Read the model definition and answer for the solid it produces. Units are mm, in the model's axes. A direction names the side the tool comes from. Coordinates: 2 decimals unless noted, no trailing zeros. Order: outer loops, then holes, each group sorted by start corner. A loop starts at its lowest first (then second) coordinate and runs counter-clockwise, first axis right, second up. Notation, with made-up numbers: (-24.5, -26) - (-12.5, -26) arc R19 ccw to (-12.5, -8) - close; hole circle Ø5 at (-23.75, 16.5). An arc over 180 degrees is marked (long way). Use one line per item in the form item = value. Start each with the question number.
from build123d import *

# Parameters (mm, degrees)
F0_R     = 10
F0_R_2   = 6
F1_DEPTH = 4
F0_R_3   = 4.15
F0_R_4   = 2.55
F2_DEPTH = 10.5
F3_DEPTH = 4.5
F4_R     = 8.5
F4_R_2   = 6
F5_DEPTH = 1.5
F7_R     = 1
F8_DEPTH = 0.2


# Not quite as in the source:
# - a fillet or chamfer that OpenCascade refuses, or shapes differently, is made with other operations: its cross-section is extruded or revolved along the edge and cut away or added
# - a feature names something its author has since deleted; it is built from what else it names


with BuildPart() as f1:
    # F0 (on Top) → F1 (new body)
    with BuildSketch(Plane.XY):
        Circle(F0_R)
        Circle(F0_R_2, mode=Mode.SUBTRACT)
    extrude(amount=F1_DEPTH)



with BuildPart() as f1b:
    # F0 (on Top) → F1, piece 2 (new body)
    with BuildSketch(Plane.XY):
        Circle(F0_R_3)
        Circle(F0_R_4, mode=Mode.SUBTRACT)
        Circle(F0_R_4)
    extrude(amount=F1_DEPTH)

    # F0 (on Top) → F2 (join)
    with BuildSketch(Plane.XY):
        Circle(F0_R_3)
        Circle(F0_R_4, mode=Mode.SUBTRACT)
    extrude(amount=F2_DEPTH)


with BuildPart() as f1_1:
    add(f1.part)

    add(f1b.part)  # F3 merges F1b
    # F0 (on Top) → F3 (join)
    with BuildSketch(Plane.XY):
        Circle(F0_R_2)
        Circle(F0_R_3, mode=Mode.SUBTRACT)
    extrude(amount=F3_DEPTH)

    # F4 (on face) → F5 (cut)
    with BuildSketch(Plane.XY):
        Circle(F4_R)
        Circle(F4_R_2, mode=Mode.SUBTRACT)
        Circle(F4_R_2)
    extrude(amount=F5_DEPTH, mode=Mode.SUBTRACT)

    # F6: fillet of radius 20 on 1 edges, made by hand

    # F6_s1 → F6_t2 (revolve)
    with BuildSketch(Plane.XZ):
        with BuildLine():
            ThreePointArc((8.5, 0), (4.7736412694, 1.1214168703), (0.9006579232, 1.5))
            Line((0.9006579232, 1.5), (8.5, 1.5))
            Line((8.5, 1.5), (8.5, 0))
        make_face()
    revolve(axis=Axis((0, 0, 1.5), (0, 0, 1)))

    # F7
    f7_edges = [f1_1.edges().sort_by_distance(p)[0] for p in [
        (-10, 0, 0),
    ]]
    fillet(f7_edges, radius=F7_R)

    # F8 (cut): a face of the model
    f8_faces = [f1_1.faces().sort_by_distance(p)[0] for p in [
        (-9.7171572875, 0, 4),
    ]]
    extrude(f8_faces, amount=-F8_DEPTH, mode=Mode.SUBTRACT)


solid = f1_1.part
Q1. For a pull along Y with two mould halves and no side action, classify faces 1 (the flat face through (0, 0, 4)), 2 (the flat face through (-2, -2, 10.5)), 3 (the cylindrical face through (-0.9, -4.05, 7.46)) as +Y half, -Y half, draft (parallel to the pull), parting line (faces both ways), or undercut.
Q2. A cutting plane is placed at B-B (z = 1.75). Give the vertices of the cut face in (x, y).
Q3. Consider probe 1 along Y at (x, z) = (0, 8.25); probe 2 along X at (y, z) = (-0.25, 3.75); probe 3 along Z at (x, y) = (-4, 3.5). Determine where each line is inside the solid, lowest interval first.
Q4. Given P1, Ø10, axis at x = -3, y = -3, coming from the +Z side; P2, Ø5, axis at x = -4.5, y = -3.5, coming from the -Z side; P3, Ø1.5, axis at x = -2, z = 4.5, coming from the -Y side; P4, Ø0.5, axis at x = -0.5, y = 0.5, coming from the -Z side, each flat-ended and moving along its own axis, determine where each tip first touches the part or whether it passes through.
Q5. A cutting plane is placed at A-A (z = 8.25). Give the vertices of the cut face in (x, y), then the cut area to 3 significant figures.
Q6. Which of the six approach directions +Z, -Z, +X, -X, +Y, -Y give full straight-line access (tool end or side, diameter ignored) to faces 4 (the flat face through (0, 0, 1.5)), 5 (the cylindrical face through (1.18, -2.26, 7.2)), 6 (the cylindrical face through (-2.17, -9.76, 2.38))?
Result sheet:
q1.face_1 = undercut
q1.face_2 = draft
q1.face_3 = parting line
q2.outline = circle Ø20 at (0, 0)
q3.probe_1 = -4.15 to -2.55, 2.55 to 4.15
q3.probe_2 = -10 to 10
q3.probe_3 = 1.01 to 4.5
q4.P1 = 10.5
q4.P2 = 0.12
q4.P3 = -9.85
q4.P4 = 1.5
q5.outline = circle Ø8.3 at (0, 0); hole circle Ø5.1 at (0, 0)
q5.area = 33.7 mm^2
q6.face_4 = -Z
q6.face_5 = +Z
q6.face_6 = +Z, -Z
